from build123d import *

# Parameters (mm, degrees)
BOSS_EXTRUDE1_DEPTH = 40
SKETCH2_R           = 6
CUT_EXTRUDE1_DEPTH  = 395
SKETCH3_R           = 5
BOSS_EXTRUDE2_DEPTH = 50


with BuildPart() as part:
    # Sketch1 → Boss-Extrude1 (new body)
    with BuildSketch(Plane(origin=(0, 0, 0), x_dir=(1, 0, 0), z_dir=(0, 1, 0))):
        Polygon((0, 170), (180, 170), (180, 130), (40, 130), (40, -130), (180, -130), (180, -170), (0, -170), align=None)
    extrude(amount=BOSS_EXTRUDE1_DEPTH)

    # Sketch2 → Cut-Extrude1 (cut)
    with BuildSketch(Plane.XY.offset(170)):
        with Locations((110, 20)):
            Circle(SKETCH2_R)
    extrude(amount=-CUT_EXTRUDE1_DEPTH, mode=Mode.SUBTRACT)

    # Sketch3 → Boss-Extrude2 (add)
    with BuildSketch(Plane(origin=(180, 0, 0), x_dir=(0, 0, -1), z_dir=(1, 0, 0))):
        with Locations(Location((-150, 20, 0), (0, 0, 180))):
            Circle(SKETCH3_R)
        with Locations(Location((150, 20, 0), (0, 0, 180))):
            Circle(SKETCH3_R)
    extrude(amount=BOSS_EXTRUDE2_DEPTH)


solid = part.part
Read the model definition and answer for the solid it produces. Units are mm, in the model's axes. A direction names the side the tool comes from. Give positions to 0.01 mm unless a question says otherwise; leave off trailing zeros. Write each loop counter-clockwise with the first axis right and the second up, starting at its lowest first coordinate (ties: lowest second). Pieces come first, ordered by that corner, then holes. Notation, with made-up numbers: (63.25, -34) -> (78.25, -34) arc R31 ccw to (78.25, 5) -> close; hole circle Ø2 at (8.25, 49.5). An arc over 180 degrees is marked (long way). Answer as a JSON object with one key per item and string values. Group by question number.
1) Find section A-A (x = 110). Write down the section's boundary in (y, z).
2) The mould has two halves that part along Z. Classify faces 1 (the flat face through (89, 20, -170)), 2 (the flat face through (109, 11, 130)), 3 (the cylindrical face through (104, 20, -150)): +Z half, -Z half, draft (parallel to the pull), parting line (faces both ways), or undercut.
3) Find section C-C (z = 150). Write down the section's boundary in (x, y).
4) A tool of negligible diameter and unlimited length cuts with its end or side. For faces 4 (the flat face through (180, 15, -146)), 5 (the flat face through (40, 20, -2)), 6 (the flat face through (31, 0, -2)), from which of +Z, -Z, +X, -X, +Y, -Y can it reach the whole face along a straight path? Write none if from no direction.
5) Find section B-B (y = 20). Write down the section's boundary in (x, z), and give its area (3 significant figures).
6) Each of these flat-tipped pins is pushed along its axis until it touches: P1, Ø12, axis at y = 18.5, z = -50, coming from the +X side; P2, Ø9.5, axis at x = 110, y = 20, coming from the +Z side. Where does it stop, or does it pass through?
7) Consider L1, parallel to Y at x = 110, z = -142; L2, parallel to Z at x = 82.5, y = 14.5; L3, parallel to X at y = 18, z = -67.5. Determine where each line is inside the solid, lowest interval first. Write a range as from..to.
8) Find section D-D (x = 196.5). Write down the section's boundary in (y, z), and give its area (3 significant figures).
Values follow:
{
 "1": {"outline": "(0, -170) -> (14, -170) -> (14, -130) -> (0, -130) -> close; (0, 130) -> (14, 130) -> (14, 170) -> (0, 170) -> close; (26, -170) -> (40, -170) -> (40, -130) -> (26, -130) -> close; (26, 130) -> (40, 130) -> (40, 170) -> (26, 170) -> close"},
 "2": {"face 1": "-Z half", "face 2": "undercut", "face 3": "draft"},
 "3": {"outline": "(0, 0) -> (180, 0) -> (180, 15) -> (230, 15) -> (230, 25) -> (180, 25) -> (180, 40) -> (0, 40) -> close; hole circle Ø12 at (110, 20)"},
 "4": {"face 4": "+X", "face 5": "+X, +Y, -Y", "face 6": "+Z, -Z, +X, -X, -Y"},
 "5": {"outline": "(0, -170) -> (104, -170) -> (104, -130) -> (40, -130) -> (40, 130) -> (104, 130) -> (104, 170) -> (0, 170) -> close; (116, -170) -> (180, -170) -> (180, -155) -> (230, -155) -> (230, -145) -> (180, -145) -> (180, -130) -> (116, -130) -> close; (116, 130) -> (180, 130) -> (180, 145) -> (230, 145) -> (230, 155) -> (180, 155) -> (180, 170) -> (116, 170) -> close", "area": "24,800 mm2"},
 "6": {"P1": "stops at x = 40", "P2": "passes through"},
 "7": {"L1": "y = 0..14, 26..40", "L2": "z = -170..-130, 130..170", "L3": "x = 0..40"},
 "8": {"outline": "circle Ø10 at (20, -150); circle Ø10 at (20, 150)", "area": "157 mm2"}
}
